from build123d import *

# Parameters (mm, degrees)
F1_W     = 70.157
F1_H     = 26.8
F2_DEPTH = 1
F0_W     = 70.157
F0_H     = 13.8
F0_R     = 3.9
F0_H_2   = 3
F3_DEPTH = 2
F0_H_3   = 10
F4_DEPTH = 1.6


with BuildPart() as f2:
    # F1 (on Top) → F2 (new body)
    with BuildSketch(Plane.XY):
        with Locations((0, 6.5)):
            Rectangle(F1_W, F1_H)
    extrude(amount=-F2_DEPTH)

    # F0 (on Top) → F3 (join)
    with BuildSketch(Plane.XY):
        Rectangle(F0_W, F0_H)
        with Locations((-28.1785, 0)):
            Circle(F0_R, mode=Mode.SUBTRACT)
        with Locations((28.1785, 0)):
            Circle(F0_R, mode=Mode.SUBTRACT)
        with Locations((0, 18.4)):
            Rectangle(F0_W, F0_H_2)
    extrude(amount=F3_DEPTH)

    # F0 (on Top) → F4 (join)
    with BuildSketch(Plane.XY):
        with Locations((0, 11.9)):
            Rectangle(F0_W, F0_H_3)
    extrude(amount=F4_DEPTH)


solid = f2.part
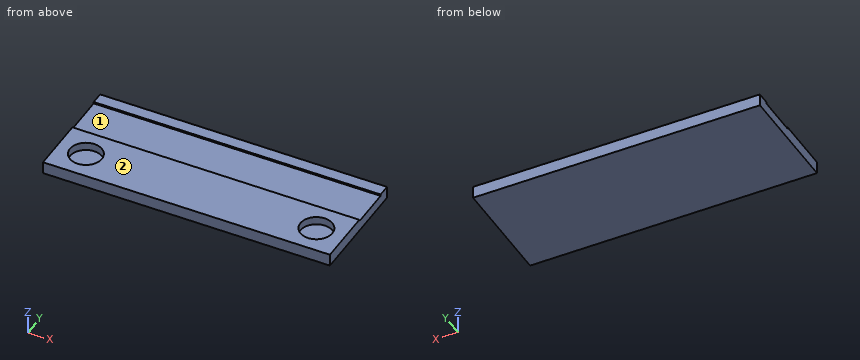
The listing builds one solid part. Answer for the finished solid, in the listing's coordinates (mm). Face numbers are marked on the shaded views. Coordinates: 2 decimals unless noted, no trailing zeros. Loops run counter-clockwise (first coordinate to the right, second up) from the corner with the lowest first, then second, coordinate; pieces in that order, holes last. Notation, with made-up numbers: (41.5, -31) -> (52.5, -31) arc R19 cw to (52.5, -5) -> close; hole circle Ø6 at (54.25, 32). An arc over 180 degrees is marked (long way). Answer in a Markdown table with one row per item. Add a question column.
1. Determine the mould class of the marked faces 1 and 2 for opening direction Y: +Y half, -Y half, draft (parallel to the pull), parting line (faces both ways), or undercut.
2. The part is cut by section D-D, the plane x = -26.5. Write down the section's boundary in (y, z), then the cut area to 3 significant figures.
3. The part is cut by section C-C, the plane z = 1.1. Write down the section's boundary in (x, y), then the cut area to 3 significant figures.
4. The part is cut by section A-A, the plane y = 0. Write down the section's boundary in (x, z), then the cut area to 3 significant figures.
5. The part is cut by section B-B, the plane x = 10.5. Write down the section's boundary in (y, z), then the cut area to 3 significant figures.
6. Consider line 1 (Y direction, x = -22.5, z = 1.85); line 2 (X direction, y = -2.25, z = 0.3); line 3 (X direction, y = 2.5, z = 0.3). Determine where each line is inside the solid, lowest interval first. Write a range as [from, to].
Answer below:
| question | item | result |
|---|---|---|
| 1 | face 1 | undercut |
| 1 | face 2 | draft |
| 2 | outline | (-6.9, -1) -> (19.9, -1) -> (19.9, 2) -> (16.9, 2) -> (16.9, 1.6) -> (6.9, 1.6) -> (6.9, 2) -> (3.52, 2) -> (3.52, 0) -> (-3.52, 0) -> (-3.52, 2) -> (-6.9, 2) -> close |
| 2 | area | 62.3 mm2 |
| 3 | outline | (-35.08, -6.9) -> (35.08, -6.9) -> (35.08, 19.9) -> (-35.08, 19.9) -> close; hole circle Ø7.8 at (-28.18, 0); hole circle Ø7.8 at (28.18, 0) |
| 3 | area | 1,780 mm2 |
| 4 | outline | (-35.08, -1) -> (35.08, -1) -> (35.08, 2) -> (32.08, 2) -> (32.08, 0) -> (24.28, 0) -> (24.28, 2) -> (-24.28, 2) -> (-24.28, 0) -> (-32.08, 0) -> (-32.08, 2) -> (-35.08, 2) -> close |
| 4 | area | 179 mm2 |
| 5 | outline | (-6.9, -1) -> (19.9, -1) -> (19.9, 2) -> (16.9, 2) -> (16.9, 1.6) -> (6.9, 1.6) -> (6.9, 2) -> (-6.9, 2) -> close |
| 5 | area | 76.4 mm2 |
| 6 | line 1 | [-6.9, 6.9], [16.9, 19.9] |
| 6 | line 2 | [-35.08, -31.36], [-24.99, 24.99], [31.36, 35.08] |
| 6 | line 3 | [-35.08, -31.17], [-25.19, 25.19], [31.17, 35.08] |
